```python
from build123d import *

# Parameters (mm, degrees)
F0_R     = 6.25
F1_DEPTH = 25


with BuildPart() as f1:
    # F0 (on Top) → F1 (new body)
    with BuildSketch(Plane.XY):
        with BuildLine():
            ThreePointArc((-50.053764, -22.16398), (-45.660366, -32.770582), (-35.053764, -37.16398))
            Line((-35.053764, -37.16398), (24.946236, -37.16398))
            ThreePointArc((24.946236, -37.16398), (35.552838, -32.770582), (39.946236, -22.16398))
            ThreePointArc((39.946236, -22.16398), (35.552838, -11.557379), (24.946236, -7.16398))
            Line((24.946236, -7.16398), (4.946236, -7.16398))
            Line((4.946236, -7.16398), (4.946236, -12.16398))
            Line((4.946236, -12.16398), (-15.053764, -12.16398))
            Line((-15.053764, -12.16398), (-15.053764, -7.16398))
            Line((-15.053764, -7.16398), (-35.053764, -7.16398))
            ThreePointArc((-35.053764, -7.16398), (-45.660366, -11.557379), (-50.053764, -22.16398))
        make_face()
        with Locations((-35.053764, -22.16398)):
            Circle(F0_R, mode=Mode.SUBTRACT)
        with Locations((24.946236, -22.16398)):
            Circle(F0_R, mode=Mode.SUBTRACT)
    extrude(amount=F1_DEPTH)


solid = f1.part
```
Read the model definition and answer for the solid it produces. Units are mm, in the model's axes. A direction names the side the tool comes from. Coordinates: 2 decimals unless noted, no trailing zeros. Write each loop counter-clockwise with the first axis right and the second up, starting at its lowest first coordinate (ties: lowest second). Pieces come first, ordered by that corner, then holes. Notation, with made-up numbers: (72.5, -0.5) - (76.5, -0.5) arc R28 ccw to (76.5, 36.5) - close; hole circle Ø1 at (17, 49). An arc over 180 degrees is marked (long way). Answer as a JSON object with one key per item and string values. Group by question number.
1. A cutting plane is placed at D-D (x = -6). Determine the outline of the cut face in (y, z).
2. Each of these flat-tipped pins is pushed along its axis until it touches: P1, Ø4, axis at y = -27.5, z = 11, coming from the +X side; P2, Ø3, axis at x = -3.5, y = -34, coming from the -Z side; P3, Ø1, axis at y = -32, z = 22, coming from the -X side; P4, Ø1.5, axis at y = -10.5, z = 4.5, coming from the +X side. Where does it stop, or does it pass through?
3. A cutting plane is placed at C-C (y = -9). Determine the outline of the cut face in (x, z), plus the area to 3 significant figures.
4. A cutting plane is placed at A-A (x = -32.5). Determine the outline of the cut face in (y, z), plus the area to 3 significant figures.
5. Consider L1, parallel to X at y = -22.5, z = 16.25; L2, parallel to X at y = -25, z = 23.75; L3, parallel to Y at x = -10, z = 1.5. Determine where each line is inside the solid, lowest interval first. Write a range as [from, to].
6. A cutting plane is placed at B-B (z = 10.5). Determine the outline of the cut face in (x, y).
7. Which of the six approach directions +Z, -Z, +X, -X, +Y, -Y give full straight-line access (tool end or side, diameter ignored) to faces 3 (the flat face through (-5, -12.164, 12)), 4 (the flat face through (-5, -37.164, 12))?
8. The mould has two halves that part along X. Classify faces 1 (the flat face through (-6, -22, 0)), 2 (the cylindrical face through (-29.3, -24.6, 12.3)): +X half, -X half, draft (parallel to the pull), parting line (faces both ways), or undercut.
Worked out:
{
 "1": {"outline": "(-37.16, 0) - (-12.16, 0) - (-12.16, 25) - (-37.16, 25) - close"},
 "2": {"P1": "stops at x = 39.57", "P2": "stops at z = 0", "P3": "stops at x = -46.79", "P4": "stops at x = 35.24"},
 "3": {"outline": "(-42.24, 0) - (-15.05, 0) - (-15.05, 25) - (-42.24, 25) - close; (4.95, 0) - (32.14, 0) - (32.14, 25) - (4.95, 25) - close", "area": "1,360 mm²"},
 "4": {"outline": "(-37.16, 0) - (-27.87, 0) - (-27.87, 25) - (-37.16, 25) - close; (-16.46, 0) - (-7.16, 0) - (-7.16, 25) - (-16.46, 25) - close", "area": "465 mm²"},
 "5": {"L1": "x = [-50.05, -41.29], [-28.81, 18.71], [31.19, 39.94]", "L2": "x = [-49.78, -40.62], [-29.48, 19.38], [30.52, 39.68]", "L3": "y = [-37.16, -12.16]"},
 "6": {"outline": "(-50.05, -22.16) arc R15 ccw to (-35.05, -37.16) - (24.95, -37.16) arc R15 ccw to (39.95, -22.16) arc R15 ccw to (24.95, -7.16) - (4.95, -7.16) - (4.95, -12.16) - (-15.05, -12.16) - (-15.05, -7.16) - (-35.05, -7.16) arc R15 ccw to start; hole circle Ø12.5 at (-35.05, -22.16); hole circle Ø12.5 at (24.95, -22.16)"},
 "7": {"face 3": "+Z, -Z, +Y", "face 4": "+Z, -Z, +X, -X, -Y"},
 "8": {"face 1": "draft", "face 2": "undercut"}
}
